Answer from the drawing. Dimensions are ordinates in mm from the lowest x, y and z of the part. A direction names the side the tool comes from. Give positions to 0.01 mm unless a question says otherwise; leave off trailing zeros. Write each loop counter-clockwise with the first axis right and the second up, starting at its lowest first coordinate (ties: lowest second). Pieces come first, ordered by that corner, then holes.
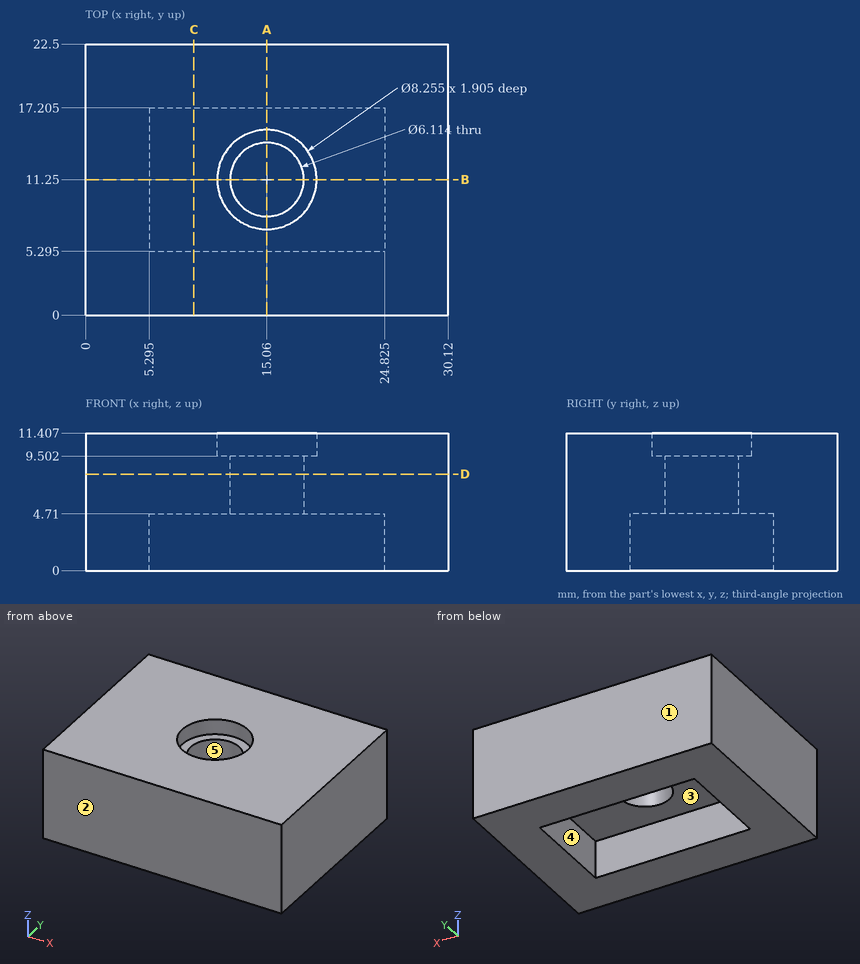
Item 1: Section C-C (x = 9) is taken. Write down the section's boundary in (y, z) (3 decimals), and give its area (3 significant figures).
Result set:
outline: (0, 0) - (5.295, 0) - (5.295, 4.71) - (17.205, 4.71) - (17.205, 0) - (22.5, 0) - (22.5, 11.407) - (0, 11.407) - close
area: 201 mm2
Item 2: Section A-A (x = 15.06) is taken. Write down the section's boundary in (y, z) (1 decimal).
Result set:
outline: (0, 0) - (5.3, 0) - (5.3, 4.7) - (8.2, 4.7) - (8.2, 9.5) - (7.1, 9.5) - (7.1, 11.4) - (0, 11.4) - close; (14.3, 4.7) - (17.2, 4.7) - (17.2, 0) - (22.5, 0) - (22.5, 11.4) - (15.4, 11.4) - (15.4, 9.5) - (14.3, 9.5) - close
Item 3: Each of these flat-tipped pins is pushed along its axis until it touches: pin 1 Ø5 at (x, z) = (19.5, 3.5) entering from -Y; pin 2 Ø2.5 at (x, y) = (15, 12) entering from +Z; pin 3 Ø2 at (x, y) = (9, 7.5) entering from -Z. Where does it stop, or does it pass through?
Result set:
pin 1: stops at y = 0
pin 2: passes through
pin 3: stops at z = 4.71
Item 4: Find the intervals of material crossed by line 1 along Y through (x, z) = (13, 1) (3 decimals); line 2 along X through (y, z) = (6.75, 2.75) (3 decimals); line 3 along Y through (x, z) = (15.06, 10.4), in increasing order.
Result set:
line 1: y = 0 to 5.295, 17.205 to 22.5
line 2: x = 0 to 5.295, 24.825 to 30.12
line 3: y = 0 to 7.12, 15.38 to 22.5
Item 5: Section D-D (z = 8) is taken. Write down the section's boundary in (x, y), and give its area (3 significant figures).
Result set:
outline: (0, 0) - (30.12, 0) - (30.12, 22.5) - (0, 22.5) - close; hole circle Ø6.11 at (15.06, 11.25)
area: 648 mm2
Item 6: Section B-B (y = 11.25) is taken. Write down the section's boundary in (x, z) (1 decimal), and give its area (3 significant figures).
Result set:
outline: (0, 0) - (5.3, 0) - (5.3, 4.7) - (12, 4.7) - (12, 9.5) - (10.9, 9.5) - (10.9, 11.4) - (0, 11.4) - close; (18.1, 4.7) - (24.8, 4.7) - (24.8, 0) - (30.1, 0) - (30.1, 11.4) - (19.2, 11.4) - (19.2, 9.5) - (18.1, 9.5) - close
area: 207 mm2
Item 7: Which of the six approach directions +Z, -Z, +X, -X, +Y, -Y give full straight-line access (tool end or side, diameter ignored) to the marked faces 4 and 5?
Result set:
face 4: -Z
face 5: +Z, -Z
Item 8: Determine the mould class of the marked faces 1, 2 and 3 for opening direction Y: pulls with the +Y half, pulls with the -Y half, needs draft (parallel to the pull), parting line crosses it, or undercut.
Result set:
face 1: pulls with the +Y half
face 2: pulls with the -Y half
face 3: undercut
